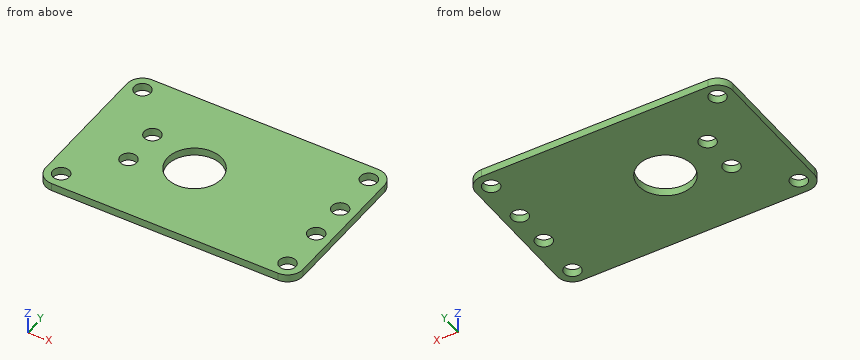
Autodesk Inventor part; units mm, degrees
ref_plane "YZ Plane" through (0, 0, 0) normal (1, 0, 0) x (0, 1, 0)
ref_plane "XZ Plane" through (0, 0, 0) normal (0, 1, 0) x (-1, 0, 0)
ref_plane "XY Plane" through (0, 0, 0) normal (0, 0, 1) x (1, 0, 0)
sketch "スケッチ1" plane through (0, 0, 0) normal (0, 0, 1) x (1, 0, 0)
  line L0 (-38, -21) -> (28.6, -21)
  line L1 (28.6, -21) -> (28.6, 21)
  line L2 (28.6, 21) -> (-38, 21)
  line L3 (-38, 21) -> (-38, -21)
  point P0 (0, 0)
  dimension "d1" = 42
  dimension "d28" = 38
  dimension "d29" = 28.6
  dimension "d32" = 21
extrude "プレート1" add sketch "スケッチ1" along normal blind 2
sketch "スケッチ2" plane through (0, 0, 2) normal (0, 0, 1) x (1, 0, 0)
  line L0 (-24, -5) -> (24.6, -5)
  line L1 (24.6, -5) -> (24.6, 5)
  line L2 (24.6, 5) -> (-24, 5)
  line L3 (-24, 5) -> (-24, -5)
  line L4 (-24, -5) -> (24.6, 5) construction
  line L5 (24.6, -5) -> (-24, 5) construction
  line L6 (28.6, -21) -> (-38, -21)
  line L7 (-38, -21) -> (-38, 21)
  line L8 (28.6, -21) -> (-38, -21)
  line L9 (28.6, 21) -> (28.6, -21)
  line L10 (-38, 21) -> (28.6, 21)
  circle A0 centre (-10, 0) radius 7
  point P0 (0.3, 0)
  point P1 (0.3, 0)
  point P2 (0.3, 0)
  point P3 (0, 0)
  dimension "d3" = 48.6
  dimension "d5" = 10
  dimension "d16" = 14
  dimension "d31" = 14
  dimension "d33" = 4
  dimension "d34" = 0
hole "穴1" at (24.6, 5, 2) at (24.6, -5, 2) at (-24, 5, 2) at (-24, -5, 2) direction (0, 0, -1) diameter 4.3 end through all
extrude "押し出し1" cut sketch "スケッチ2" against normal blind 10 contours A0 L2 L0 | L0 A0 | A0 L2
sketch "スケッチ3" plane through (0, 0, 2) normal (0, 0, 1) x (1, 0, 0)
  line L0 (-38, 21) -> (28.6, 21)
  line L1 (-38, -21) -> (-38, 21)
  line L2 (28.6, -21) -> (-38, -21)
  line L3 (28.6, 21) -> (28.6, -21)
  line L4 (24.6, 17) -> (-34, 17)
  line L5 (-34, 17) -> (-34, -17)
  line L6 (-34, -17) -> (24.6, -17)
  line L7 (24.6, -17) -> (24.6, 17)
  point P0 (0, 0)
  dimension "d19" = 4
hole "穴2" at (-34, 17, 2) at (-34, -17, 2) at (24.6, 17, 2) at (24.6, -17, 2) direction (0, 0, -1) diameter 4.3 end through all
fillet "コーナーR1" radius 4 4 edges at (28.6, 21, 1) (-38, 21, 1) (-38, -21, 1) (28.6, -21, 1)
equation "\"d14\" = Thickness"
equation "\"d2\" = Thickness"
equation "\"BendRadius\" = Thickness"
equation "\"BendReliefWidth\" = Thickness"
equation "\"BendReliefDepth\" = 0.5 * Thickness"
equation "\"CornerReliefSize\" = 4 * Thickness"
equation "\"MinimumRemnant\" = 2 * Thickness"
equation "\"TransitionRadius\" = BendRadius"
equation "\"JacobiRadiusSize\" = BendRadius"
equation "\"GapSize\" = Thickness"
properties part number "s_carbon_plate8" material "CFRP"
Read the model definition and answer for the solid it produces. Units are mm, in the model's axes. Round coordinates to 2 decimals unless told otherwise and drop trailing zeros. Write each loop counter-clockwise with the first axis right and the second up, starting at its lowest first coordinate (ties: lowest second). Pieces come first, ordered by that corner, then holes.
1. Given pin 1 Ø4 at (x, y) = (24.6, -17) entering from -Z, flat-ended and moving along its own axis, determine where the tip first touches the part or whether it passes through.
2. The part is cut by section C-C, the plane y = -5. Determine the outline of the cut face in (x, z).
3. The part is cut by section D-D, the plane x = -24. Determine the outline of the cut face in (y, z), then the cut area to 3 significant figures.
4. The part is cut by section B-B, the plane x = -10. Determine the outline of the cut face in (y, z).
5. The part is cut by section A-A, the plane z = 0.3. State how many separate pieces and enclosed holes the cut face has, then the cut area to 3 significant figures.
6. Straight lines are drawn through the part: L1, parallel to Y at x = -34, z = 1.6; L2, parallel to X at y = 17, z = 1.65; L3, parallel to X at y = 0, z = 1.25. For each, find the intervals that lie inside material, in ascending order.
Values:
1. pin 1: passes through
2. outline: (-38, 0) - (-26.15, 0) - (-26.15, 2) - (-38, 2) - close; (-21.85, 0) - (-14.9, 0) - (-14.9, 2) - (-21.85, 2) - close; (-5.1, 0) - (22.45, 0) - (22.45, 2) - (-5.1, 2) - close; (26.75, 0) - (28.6, 0) - (28.6, 2) - (26.75, 2) - close
3. outline: (-21, 0) - (-7.15, 0) - (-7.15, 2) - (-21, 2) - close; (-2.85, 0) - (2.85, 0) - (2.85, 2) - (-2.85, 2) - close; (7.15, 0) - (21, 0) - (21, 2) - (7.15, 2) - close
3. area: 66.8 mm2
4. outline: (-21, 0) - (-7, 0) - (-7, 2) - (-21, 2) - close; (7, 0) - (21, 0) - (21, 2) - (7, 2) - close
5. separate pieces: 1
5. enclosed holes: 9
5. area: 2,510 mm2
6. L1: y = -21 to -19.15, -14.85 to 14.85, 19.15 to 21
6. L2: x = -38 to -36.15, -31.85 to 22.45, 26.75 to 28.6
6. L3: x = -38 to -17, -3 to 28.6
